Could you check a few things on this drawing? It's one solid part, dimensions in mm from its lowest x, y, z. Round coordinates to 2 decimals unless told otherwise and drop trailing zeros. Write each loop counter-clockwise with the first axis right and the second up, starting at its lowest first coordinate (ties: lowest second). Pieces come first, ordered by that corner, then holes. Notation, with made-up numbers: (6.5, -37) -> (17.5, -37) arc R25 ccw to (17.5, -1) -> close; hole circle Ø9 at (64, 40.5). An arc over 180 degrees is marked (long way). Put each result on its own line as item: value. Start each with the question number.
1) Will this pin go through, and if not, where does the flat tip stop? P1, Ø1, axis at x = 1, y = 2, coming from the +Z side.
2) I want a section at B-B, the plane z = 5.25. List the corners of the cut face in (x, y) for me (1 decimal), then the cut area to 3 significant figures.
3) I want a section at A-A, the plane x = 4.25. List the corners of the cut face in (y, z) for me.
4) We'd pull the mould along Z, two halves only. Please class the marked faces 1, 2 and 3: released by +Z, released by -Z, zero draft, split by the parting line, or undercut.
5) If I drill on line 1 along X through (y, z) = (2.7, 3) (1 decimal); line 2 along Z through (x, y) = (3, 1.2); line 3 along Z through (x, y) = (3.5, 0.2), over which ranges is the centre line in solid material (lowest first)? Write a range as [from, to].
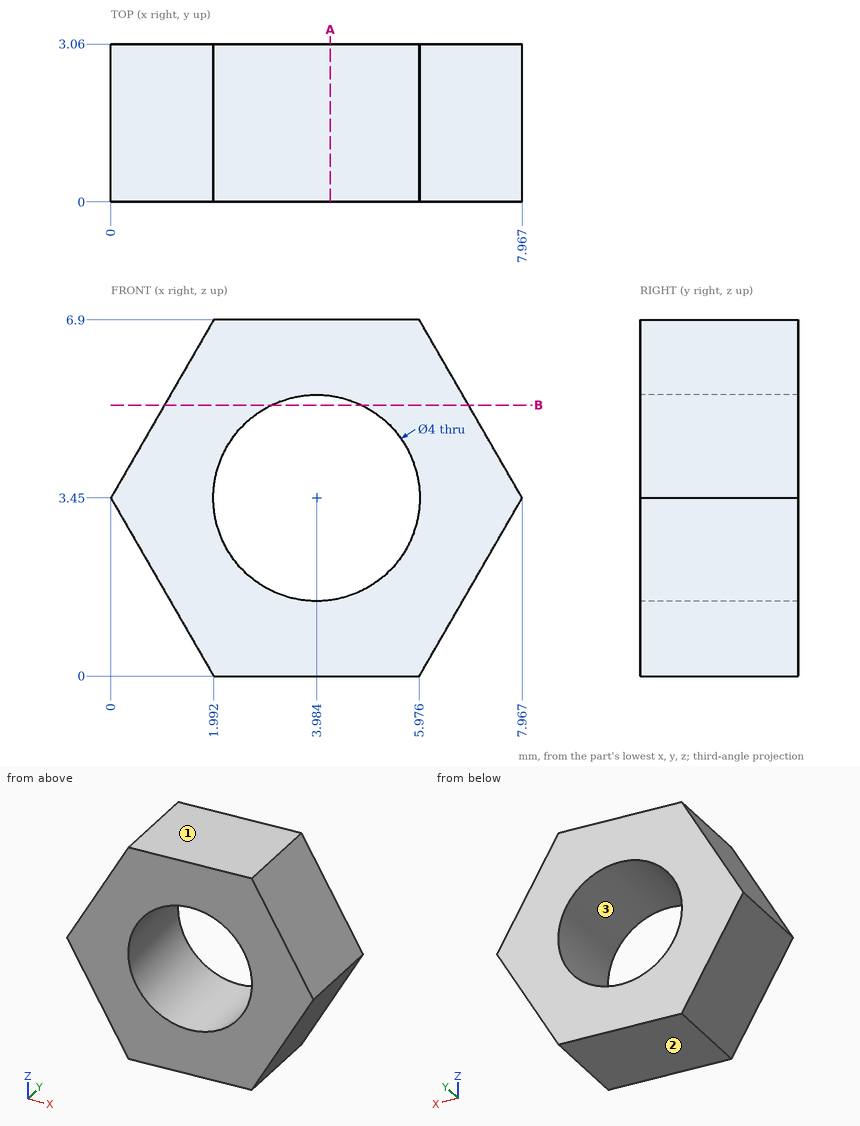
Findings:
1. P1: stops at z = 6.05
2. outline: (1, 0) -> (3.1, 0) -> (3.1, 3.1) -> (1, 3.1) -> close; (4.9, 0) -> (6.9, 0) -> (6.9, 3.1) -> (4.9, 3.1) -> close
2. area: 12.7 mm2
3. outline: (0, 0) -> (3.06, 0) -> (3.06, 1.47) -> (0, 1.47) -> close; (0, 5.43) -> (3.06, 5.43) -> (3.06, 6.9) -> (0, 6.9) -> close
4. face 1: released by +Z
4. face 2: released by -Z
4. face 3: undercut
5. line 1: x = [0.3, 2], [5.9, 7.7]
5. line 2: z = [0, 1.71], [5.19, 6.9]
5. line 3: z = [0, 1.51], [5.39, 6.9]
